Input: part model. Units: mm. Frame: model coordinates. A direction names the side the tool comes from. Give positions to 0.01 mm unless a question says otherwise; leave off trailing zeros. Write each loop counter-clockwise with the first axis right and the second up, starting at its lowest first coordinate (ties: lowest second). Pieces come first, ordered by that corner, then holes. Notation, with made-up numbers: (51.25, 85.5) -> (71.25, 85.5) arc R31 ccw to (71.25, 118.5) -> close; hole circle Ø6 at (-28.75, 34). An arc over 180 degrees is marked (long way). Return JSON: item names as keys, results as strings. Group by question number.
Item 1: Pin query (flat end, axial travel): P1, Ø12, axis at x = 121.5, z = -3, coming from the +Y side; P2, Ø6, axis at x = 100.5, z = -5, coming from the +Y side; P3, Ø3, axis at x = 82, y = -12, coming from the -Z side. Return the tip coordinate at first contact, or that it passes through.
Item 2: Section B-B, the plane x = 86.5. Return loops of the section in (y, z).
Item 3: Mould query, pull axis X, two halves, no side actions, for faces 5 (the face through (0, 0, 0)), 6 (the face through (139, 0, 0)), 7 (the face through (8.1, -3, 16)), 8 (the face through (4.6, -13.887, -10.648)). Classes: released by +X, released by -X, zero draft, split by the parting line, or undercut.
Item 4: Section A-A, the plane x = 46.5. Return loops of the section in (y, z), then the cut area to 3 significant figures.
Item 5: Set-up query: faces 1 (the face through (9.06, -12.54, -9.61)), 2 (the face through (37, 9.9, -18.2)), 3 (the face through (21.154, -13.887, -10.648)), 4 (the face through (34.535, 10.382, -19.961)). Return all of +Z, -Z, +X, -X, +Y, -Y with unobstructed straight access to the full face (end or side cutting, diameter ignored); none if empty.
Item 6: Line query: line 1 (Y direction, x = 22, z = 0.5); line 2 (Z direction, x = 50, y = -1); line 3 (X direction, y = 9.5, z = 16.5). Output: solid intervals per line, ascending. Write a range as [from, to].
Autodesk Inventor part; units mm, degrees
ref_plane "YZ Plane" through (0, 0, 0) normal (1, 0, 0) x (0, 1, 0)
ref_plane "XZ Plane" through (0, 0, 0) normal (0, 1, 0) x (-1, 0, 0)
ref_plane "XY Plane" through (0, 0, 0) normal (0, 0, 1) x (1, 0, 0)
sketch "Эскиз1" plane through (0, 0, 0) normal (0, 0, 1) x (1, 0, 0)
  line L0 (0, 0) -> (0, 17.5)
  line L1 (0, 17.5) -> (8.1, 17.5)
  line L2 (8.1, 17.5) -> (8.1, 15.8)
  line L3 (8.1, 15.8) -> (10, 15.8)
  line L4 (10, 15.8) -> (10, 17.5)
  line L5 (10, 17.5) -> (32, 17.5)
  line L6 (32, 17.5) -> (32, 22.5)
  line L7 (32, 22.5) -> (37, 22.5)
  line L8 (37, 22.5) -> (37, 17.5)
  line L9 (37, 17.5) -> (79, 17.5)
  line L10 (79, 17.5) -> (79, 16.5)
  line L11 (79, 16.5) -> (89, 16.5)
  line L12 (89, 16.5) -> (89, 15)
  line L13 (89, 15) -> (139, 15)
  line L14 (139, 15) -> (139, 0)
  line L15 (139, 0) -> (0, 0)
  line L16 (-27.8, 0) -> (166.8, 0) construction
  line L17 (0, -4.5) -> (0, 27) construction
  point P0 (0, 0)
  dimension "d1" = 1.9
  dimension "d2" = 10
  dimension "d3" = 22
  dimension "d4" = 5
  dimension "d5" = 42
  dimension "d6" = 10
  dimension "d7" = 50
  dimension "d12" = 0
  dimension "d13" = 1.7
  dimension "d14" = 0
  dimension "d16" = 35
  dimension "d17" = 45
  dimension "d18" = 33
  dimension "d20" = 30
revolve "Вращение1" add sketch "Эскиз1" angle 360 about axis through (-10, 0, 0) along (1, 0, 0)
thread "Резьба1"
chamfer "Фаска1" distance 1 angle 45 1 edges at (0, -17.5, 0)
sketch "Эскиз2" plane through (0, 0, 0) normal (0, 0, 1) x (1, 0, 0)
  line L0 (37, 17.5) -> (79, 17.5) construction
  line L1 (37, -22.5) -> (37, 22.5) construction
  line L2 (37, 20.55) -> (36.7, 20.25)
  line L3 (36.7, 20.25) -> (36.7, 17.25)
  line L4 (36.7, 17.25) -> (39.7, 17.25)
  line L5 (39.7, 17.25) -> (39.95, 17.5)
  line L6 (37, 20.55) -> (39.95, 20.55)
  line L7 (39.95, 20.55) -> (39.95, 17.5)
  line L8 (-27.8, 0) -> (166.8, 0)
  point P0 (0, 0)
  dimension "d27" = 45
  dimension "d28" = 45
  dimension "d29" = 3
  dimension "d31" = 0.3
  dimension "d32" = 0.25
revolve "Вращение2" cut sketch "Эскиз2" angle 360 about axis through (-10, 0, 0) along (1, 0, 0)
fillet "Сопряжение1" radius 1 1 edges at (36.7, -17.25, 0)
fillet "Сопряжение2" radius 0.5 1 edges at (36.7, -20.25, 0)
fillet "Сопряжение3" radius 0.5 1 edges at (39.7, -17.25, 0)
properties part number "big"
Answer below:
{
 "1": {"P1": "stops at y = 15", "P2": "stops at y = 14.87", "P3": "stops at z = -12.73"},
 "2": {"outline": "circle Ø33 at (0, 0)"},
 "3": {"face 5": "released by -X", "face 6": "released by +X", "face 7": "undercut", "face 8": "zero draft"},
 "4": {"outline": "circle Ø35 at (0, 0)", "area": "962 mm2"},
 "5": {"face 1": "none", "face 2": "+X", "face 3": "-X", "face 4": "+X, -X"},
 "6": {"line 1": "y = [-17.49, 17.49]", "line 2": "z = [-17.47, 17.47]", "line 3": "x = [32, 36.7]"}
}
